from build123d import *

# Parameters (mm, degrees)
SKETCH1_R           = 2.5527
SKETCH1_R_2         = 3.3274
BOSS_EXTRUDE1_DEPTH = 533.4


with BuildPart() as part:
    # Sketch1 → Boss-Extrude1 (new body)
    with BuildSketch(Plane(origin=(0, 0, -533.4), x_dir=(-1, 0, 0), z_dir=(0, 0, -1))):
        with BuildLine():
            Line((19.05, 3.175), (19.05, 15.875))
            ThreePointArc((19.05, 15.875), (18.12006403, 18.12006403), (15.875, 19.05))
            Line((15.875, 19.05), (5.6388, 19.05))
            ThreePointArc((5.6388, 19.05), (4.525248241, 18.588751759), (4.064, 17.4752))
            Line((4.064, 17.4752), (4.064, 16.5608))
            ThreePointArc((4.064, 16.5608), (4.525248241, 15.447248241), (5.6388, 14.986))
            Line((5.6388, 14.986), (9.398, 14.986))
            ThreePointArc((9.398, 14.986), (10.026617928, 14.725617928), (10.287, 14.097))
            Line((10.287, 14.097), (10.287, 13.779435857))
            ThreePointArc((10.287, 13.779435857), (10.219328904, 13.439230286), (10.026617928, 13.150817928))
            Line((10.026617928, 13.150817928), (5.124984211, 8.249184211))
            ThreePointArc((5.124984211, 8.249184211), (3.584038188, 7.219556996), (1.766368421, 6.858))
            Line((1.766368421, 6.858), (-1.766368421, 6.858))
            ThreePointArc((-1.766368421, 6.858), (-3.584038188, 7.219556996), (-5.124984211, 8.249184211))
            Line((-5.124984211, 8.249184211), (-10.026617928, 13.150817928))
            ThreePointArc((-10.026617928, 13.150817928), (-10.219328904, 13.439230286), (-10.287, 13.779435857))
            Line((-10.287, 13.779435857), (-10.287, 14.097))
            ThreePointArc((-10.287, 14.097), (-10.026617928, 14.725617928), (-9.398, 14.986))
            Line((-9.398, 14.986), (-5.6388, 14.986))
            ThreePointArc((-5.6388, 14.986), (-4.525248241, 15.447248241), (-4.064, 16.5608))
            Line((-4.064, 16.5608), (-4.064, 17.4752))
            ThreePointArc((-4.064, 17.4752), (-4.525248241, 18.588751759), (-5.6388, 19.05))
            Line((-5.6388, 19.05), (-15.875, 19.05))
            ThreePointArc((-15.875, 19.05), (-18.12006403, 18.12006403), (-19.05, 15.875))
            Line((-19.05, 15.875), (-19.05, 3.175))
            ThreePointArc((-19.05, 3.175), (-18.12006403, 0.92993597), (-15.875, 0))
            Line((-15.875, 0), (15.875, 0))
            ThreePointArc((15.875, 0), (18.12006403, 0.92993597), (19.05, 3.175))
        make_face()
        with Locations(Location((14.848797074, 14.801432678, 0), (0, 0, 180))):
            Circle(SKETCH1_R, mode=Mode.SUBTRACT)
        with Locations(Location((12.7, 6.35, 0), (0, 0, 180))):
            Circle(SKETCH1_R_2, mode=Mode.SUBTRACT)
        with Locations(Location((-12.7, 6.35, 0), (0, 0, 180))):
            Circle(SKETCH1_R_2, mode=Mode.SUBTRACT)
        with Locations(Location((-14.848797074, 14.801432678, 0), (0, 0, 180))):
            Circle(SKETCH1_R, mode=Mode.SUBTRACT)
    extrude(amount=-BOSS_EXTRUDE1_DEPTH)


solid = part.part
Verification items for the finished model (mm, model axes). Coordinates: 2 decimals unless noted, no trailing zeros. One line per question, with ' | ' between items.
1) Sectioned sample at A-A on z = -271.5. State how many separate pieces and enclosed holes the cut face has, then the cut area to 3 significant figures.
Solutions:
separate pieces: 1 | enclosed holes: 4 | area: 449 mm^2
2) Depth check by flat-ended pin: pin 1 Ø6.5 at (x, y) = (14.85, 14.8) entering from +Z; pin 2 Ø0.5 at (y, z) = (17, -178) entering from +X; pin 3 Ø1.5 at (x, z) = (3.5, -260.5) entering from +Y; pin 4 Ø0.5 at (y, z) = (17, -372) entering from -X. Enter the tip coordinate at first touch or a pass-through.
Solutions:
pin 1: z = 0 | pin 2: x = 18.93 | pin 3: y = 18.22 | pin 4: x = -18.93
3) Material ranges on L1, parallel to X at y = 6.5, z = -34; L2, parallel to Y at x = 12, z = -264; L3, parallel to Y at x = -7, z = -89, recorded low to high.
Solutions:
L1: -19.05 to -16.02, -9.38 to 9.38, 16.02 to 19.05 | L2: 0 to 3.1, 9.6 to 19.05 | L3: 0 to 10.12, 14.99 to 19.05
